```python
from build123d import *

# Parameters (mm, degrees)
EXTRUDE_1_DEPTH                  = 296
CUT_EXTRUDE_1_REACH              = 375.122
SKETCH_2_R                       = 24
EXTRUDE_START                    = -296
EXTRUDE_2_DEPTH                  = 296
CUT_EXTRUDE_2_REACH              = 369.94
CUT_EXTRUDE_2_DIRECTION_2_REACH  = 369.94
SKETCH_5_R                       = 38
CUT_EXTRUDE_4_DEPTH              = 16
CUT_EXTRUDE_4_DIRECTION_2_REACH  = 369.94
CUT_EXTRUDE_10_REACH             = 369.94
CUT_EXTRUDE_11_REACH             = 369.94
CUT_EXTRUDE_12_REACH             = 369.94
CUT_EXTRUDE_12_DIRECTION_2_REACH = 369.94
CUT_EXTRUDE_1_2_DEPTH            = 374.122168517
CUT_EXTRUDE_1_2_DEPTH_BACK       = 6
SKETCH_10_W                      = 353.554121084
SKETCH_10_H                      = 70
CUT_EXTRUDE_2_2_DEPTH            = 374.122168517
CUT_EXTRUDE_2_2_DEPTH_BACK       = 10
SKETCH_11_W                      = 315.319296241
SKETCH_11_H                      = 70
CUT_EXTRUDE_13_DEPTH             = 49.976974814


with BuildPart() as part:
    # 草图1 → 凸台-拉伸1 (new body)
    with BuildSketch(Plane.XY):
        with BuildLine():
            Line((-75.187918949, 11.080471294), (-92, -103))
            Line((-92, -103), (-92, -153))
            Line((-92, -153), (-63, -182))
            Line((-63, -182), (-25.55454992, -183.234465387))
            Line((-25.55454992, -183.234465387), (-23.907851937, -133.284626575))
            Line((-23.907851937, -133.284626575), (27.064456588, -134.965032351))
            Line((27.064456588, -134.965032351), (25.417758605, -184.914871163))
            Line((25.417758605, -184.914871163), (109, -187.67032967))
            Line((109, -187.67032967), (128, -168.67032967))
            Line((128, -168.67032967), (128, -85.67032967))
            Line((128, -85.67032967), (87.212696765, -70.515157246))
            Line((87.212696765, -70.515157246), (75.187918949, 11.080471294))
            ThreePointArc((75.187918949, 11.080471294), (0, 76), (-75.187918949, 11.080471294))
        make_face()
    extrude(amount=EXTRUDE_1_DEPTH)

    # 草图2 → Cut-Extrude 1 (cut, up to next)
    with BuildSketch(Plane.XY.offset(296), mode=Mode.PRIVATE) as cut_extrude_1_sk1:
        Circle(SKETCH_2_R)
    cut_extrude_1_tool1 = extrude(cut_extrude_1_sk1.sketch, amount=-CUT_EXTRUDE_1_REACH, mode=Mode.PRIVATE) & part.part
    add(cut_extrude_1_tool1.solids().sort_by_distance((0, 0, 296))[0], mode=Mode.SUBTRACT)

    # 草图3 → 凸台-拉伸2 (add)
    with BuildSketch(Plane.XY.offset(296).offset(EXTRUDE_START)):
        with BuildLine():
            Line((54, 53.478967828), (54, 166))
            Line((54, 166), (16, 166))
            Line((16, 166), (16, 120))
            Line((16, 120), (-12.175135195, 75.018438287))
            ThreePointArc((-12.175135195, 75.018438287), (23.522691723, 72.268132494), (54, 53.478967828))
        make_face()
    extrude(amount=EXTRUDE_2_DEPTH)

    # 草图4 → Cut-Extrude 2 (cut, up to next)
    with BuildSketch(Plane.ZY.offset(-16), mode=Mode.PRIVATE) as cut_extrude_2_sk1:
        with BuildLine():
            Line((159, 124), (159, 116))
            ThreePointArc((159, 116), (148, 105), (137, 116))
            Line((137, 116), (137, 124))
            ThreePointArc((137, 124), (148, 135), (159, 124))
        make_face()
    cut_extrude_2_tool1 = extrude(cut_extrude_2_sk1.sketch, amount=-CUT_EXTRUDE_2_REACH, mode=Mode.PRIVATE) & part.part
    add(cut_extrude_2_tool1.solids().sort_by_distance((16, 120, 148))[0], mode=Mode.SUBTRACT)

    # 草图4 → Cut-Extrude 2 direction 2 (cut, up to next)
    with BuildSketch(Plane.ZY.offset(-16), mode=Mode.PRIVATE) as cut_extrude_2_direction_2_sk1:
        with BuildLine():
            Line((159, 124), (159, 116))
            ThreePointArc((159, 116), (148, 105), (137, 116))
            Line((137, 116), (137, 124))
            ThreePointArc((137, 124), (148, 135), (159, 124))
        make_face()
    cut_extrude_2_direction_2_tool1 = extrude(cut_extrude_2_direction_2_sk1.sketch, amount=CUT_EXTRUDE_2_DIRECTION_2_REACH, mode=Mode.PRIVATE) & part.part
    add(cut_extrude_2_direction_2_tool1.solids().sort_by_distance((16, 120, 148))[0], mode=Mode.SUBTRACT)

    # 草图5 → 切除-拉伸4 (cut)
    with BuildSketch(Plane.ZY.offset(-16)):
        with Locations((148, 120)):
            Circle(SKETCH_5_R)
    extrude(amount=-CUT_EXTRUDE_4_DEPTH, mode=Mode.SUBTRACT)

    # 草图5 → 切除-拉伸4 direction 2 (cut, up to next)
    with BuildSketch(Plane.ZY.offset(-16), mode=Mode.PRIVATE) as cut_extrude_4_direction_2_sk1:
        with Locations((148, 120)):
            Circle(SKETCH_5_R)
    cut_extrude_4_direction_2_tool1 = extrude(cut_extrude_4_direction_2_sk1.sketch, amount=CUT_EXTRUDE_4_DIRECTION_2_REACH, mode=Mode.PRIVATE) & part.part
    add(cut_extrude_4_direction_2_tool1.solids().sort_by_distance((16, 120, 148))[0], mode=Mode.SUBTRACT)

    # 草图6 → 切除-拉伸10 (cut, up to next)
    with BuildSketch(Plane.ZY.offset(-16), mode=Mode.PRIVATE) as cut_extrude_10_sk1:
        with BuildLine():
            Line((195.958315233, 120), (296, 120))
            Line((296, 120), (296, 166))
            Line((296, 166), (148, 166))
            ThreePointArc((148, 166), (181.226495452, 152.641016151), (195.958315233, 120))
        make_face()
    cut_extrude_10_tool1 = extrude(cut_extrude_10_sk1.sketch, amount=-CUT_EXTRUDE_10_REACH, mode=Mode.PRIVATE) & part.part
    add(cut_extrude_10_tool1.solids().sort_by_distance((16, 144.191812, 240.106882))[0], mode=Mode.SUBTRACT)

    # 草图6<5> → 切除-拉伸11 (cut, up to next)
    with BuildSketch(Plane.ZY.offset(-16), mode=Mode.PRIVATE) as cut_extrude_11_sk1:
        with BuildLine():
            ThreePointArc((100.041684767, 120), (114.773504548, 152.641016151), (148, 166))
            Line((148, 166), (0, 166))
            Line((0, 166), (0, 120))
            Line((0, 120), (100.041684767, 120))
        make_face()
    cut_extrude_11_tool1 = extrude(cut_extrude_11_sk1.sketch, amount=-CUT_EXTRUDE_11_REACH, mode=Mode.PRIVATE) & part.part
    add(cut_extrude_11_tool1.solids().sort_by_distance((16, 144.191812, 55.893118))[0], mode=Mode.SUBTRACT)

    # 草图6<6> → 切除-拉伸12 (cut, up to next)
    with BuildSketch(Plane.ZY.offset(-16), mode=Mode.PRIVATE) as cut_extrude_12_sk1:
        with BuildLine():
            ThreePointArc((100.041684767, 116), (100, 118), (100.041684767, 120))
            Line((100.041684767, 120), (0, 120))
            Line((0, 120), (0, 75.018438287))
            Line((0, 75.018438287), (10, 75.018438287))
            Line((10, 75.018438287), (100.041684767, 116))
        make_face()
    cut_extrude_12_tool1 = extrude(cut_extrude_12_sk1.sketch, amount=-CUT_EXTRUDE_12_REACH, mode=Mode.PRIVATE) & part.part
    # 草图6<6> → 切除-拉伸12 (cut, up to next)
    with BuildSketch(Plane.ZY.offset(-16), mode=Mode.PRIVATE) as cut_extrude_12_sk2:
        with BuildLine():
            Line((286, 75.018438287), (296, 75.018438287))
            Line((296, 75.018438287), (296, 120))
            Line((296, 120), (195.958315233, 120))
            ThreePointArc((195.958315233, 120), (196, 118), (195.958315233, 116))
            Line((195.958315233, 116), (286, 75.018438287))
        make_face()
    cut_extrude_12_tool2 = extrude(cut_extrude_12_sk2.sketch, amount=-CUT_EXTRUDE_12_REACH, mode=Mode.PRIVATE) & part.part
    add(cut_extrude_12_tool1.solids().sort_by_distance((16, 103.644966, 36.114885))[0], mode=Mode.SUBTRACT)
    add(cut_extrude_12_tool2.solids().sort_by_distance((16, 103.644966, 259.885115))[0], mode=Mode.SUBTRACT)

    # 草图6<6> → 切除-拉伸12 direction 2 (cut, up to next)
    with BuildSketch(Plane.ZY.offset(-16), mode=Mode.PRIVATE) as cut_extrude_12_direction_2_sk1:
        with BuildLine():
            ThreePointArc((100.041684767, 116), (100, 118), (100.041684767, 120))
            Line((100.041684767, 120), (0, 120))
            Line((0, 120), (0, 75.018438287))
            Line((0, 75.018438287), (10, 75.018438287))
            Line((10, 75.018438287), (100.041684767, 116))
        make_face()
    cut_extrude_12_direction_2_tool1 = extrude(cut_extrude_12_direction_2_sk1.sketch, amount=CUT_EXTRUDE_12_DIRECTION_2_REACH, mode=Mode.PRIVATE) & part.part
    # 草图6<6> → 切除-拉伸12 direction 2 (cut, up to next)
    with BuildSketch(Plane.ZY.offset(-16), mode=Mode.PRIVATE) as cut_extrude_12_direction_2_sk2:
        with BuildLine():
            Line((286, 75.018438287), (296, 75.018438287))
            Line((296, 75.018438287), (296, 120))
            Line((296, 120), (195.958315233, 120))
            ThreePointArc((195.958315233, 120), (196, 118), (195.958315233, 116))
            Line((195.958315233, 116), (286, 75.018438287))
        make_face()
    cut_extrude_12_direction_2_tool2 = extrude(cut_extrude_12_direction_2_sk2.sketch, amount=CUT_EXTRUDE_12_DIRECTION_2_REACH, mode=Mode.PRIVATE) & part.part
    add(cut_extrude_12_direction_2_tool1.solids().sort_by_distance((16, 103.644966, 36.114885))[0], mode=Mode.SUBTRACT)
    add(cut_extrude_12_direction_2_tool2.solids().sort_by_distance((16, 103.644966, 259.885115))[0], mode=Mode.SUBTRACT)

    # 草图10 → Cut-Extrude 1 2 (cut, two sides: drawn at the far end of the back side and taken through both)
    with BuildSketch(Plane.XY.offset(296).offset(-CUT_EXTRUDE_1_2_DEPTH_BACK)):
        with Locations((35.701307798, -162)):
            Rectangle(SKETCH_10_W, SKETCH_10_H)
    extrude(amount=CUT_EXTRUDE_1_2_DEPTH + CUT_EXTRUDE_1_2_DEPTH_BACK, mode=Mode.SUBTRACT)

    # 草图11 → Cut-Extrude 2 2 (cut, two sides: drawn at the far end of the back side and taken through both)
    with BuildSketch(Plane(origin=(0, 0, 0), x_dir=(-1, 0, 0), z_dir=(0, 0, -1)).offset(-CUT_EXTRUDE_2_2_DEPTH_BACK)):
        with Locations((-8.559302508, -162)):
            Rectangle(SKETCH_11_W, SKETCH_11_H)
    extrude(amount=CUT_EXTRUDE_2_2_DEPTH + CUT_EXTRUDE_2_2_DEPTH_BACK, mode=Mode.SUBTRACT)

    # 草图12 → 切除-拉伸13 (cut)
    with BuildSketch(Plane(origin=(-6.061881785, -183.87708082, 0), x_dir=(0.9994570299138168, -0.032949132854323, 0), z_dir=(-0.032949132854323, -0.9994570299138168, 0))):
        with BuildLine():
            Line((31.496742179, 262.5), (87.843649763, 79.657100204))
            ThreePointArc((87.843649763, 79.657100204), (70.653842384, 47.153092416), (38.149834596, 64.342899796))
            Line((38.149834596, 64.342899796), (31.496742179, 85.931852273))
            Line((31.496742179, 85.931852273), (31.496742179, 262.5))
        make_face()
    extrude(amount=-CUT_EXTRUDE_13_DEPTH, mode=Mode.SUBTRACT)


solid = part.part
```
For this review, take the finished solid that the model builds, in its own axes (mm). A direction names the side the tool comes from. Coordinates: 2 decimals unless noted, no trailing zeros. Order: outer loops, then holes, each group sorted by start corner. A loop starts at its lowest first (then second) coordinate and runs counter-clockwise, first axis right, second up. Notation, with made-up numbers: (-27, 43) - (-11, 43) arc R15 cw to (-11, 48) - close; hole circle Ø2 at (-7.5, -1.75). An arc over 180 degrees is marked (long way). Answer as a JSON object with one key per item and string values. Group by question number.
1. For probe 1 along Y at (x, z) = (26, 148); probe 2 along Z at (x, y) = (-36, -154.5); probe 3 along Y at (x, z) = (0, 235), list the stretches that pass through material, from the lowest coordinate up.
2. The part is to be moulded in two halves that separate along Y. For faces 1 (the flat face through (28.73, 95.22, 54.39)), 2 (the cylindrical face through (43, 105, 148)), 3 (the flat face through (43, 120, 137)), 4 (the flat face through (128, -128, 146)), say which applies: pulls with the +Y half, pulls with the -Y half, needs draft (parallel to the pull), parting line crosses it, or undercut.
3. Clearance check with flat-ended pins moving along their axes: P1, Ø1, axis at y = 45, z = 131.5, coming from the +X side; P2, Ø2.5, axis at x = 47, y = 119.5, coming from the -Z side; P3, Ø4, axis at y = -84.5, z = 127.5, coming from the -X side; P4, Ø1.5, axis at x = -58, y = -39.5, coming from the -Z side. State where each tip first meets the part, or that it passes through.
4. We need section A-A on z = 21.5. State the section outline as (x, y) points, then the cut area to 3 significant figures.
5. For faces 5 (the flat face through (54, 84, 146)), 6 (the cylindrical face through (43, 135, 148)), 7 (the flat face through (41, -157, 290)), list the 3-axis set-ups (+Z, -Z, +X, -X, +Y, -Y) from which the entire face can be reached by the end or side of a thin tool; tool diameter is ignored.
6. We need section C-C on x = 0. State the section outline as (y, z) points, then the cut area to 3 significant figures.
7. We need section D-D on y = 97. State the section outline as (x, z) points.
8. We need section B-B on y = 0. State the section outline as (x, z) points, then the cut area to 3 significant figures.
Final values:
{
 "1": {"probe 1": "-134.93 to 82, 158 to 166", "probe 2": "10 to 290", "probe 3": "-134.07 to -24, 24 to 94.46"},
 "2": {"face 1": "pulls with the +Y half", "face 2": "undercut", "face 3": "undercut", "face 4": "needs draft"},
 "3": {"P1": "x = 61.61", "P2": "z = 100", "P3": "x = -89.57", "P4": "z = 0"},
 "4": {"outline": "(-92, -153) - (-63, -182) - (-25.55, -183.23) - (-23.91, -133.28) - (27.06, -134.97) - (25.42, -184.91) - (109, -187.67) - (128, -168.67) - (128, -85.67) - (87.21, -70.52) - (75.19, 11.08) arc R76 ccw to (54, 53.48) - (54, 80.25) - (-8.9, 80.25) - (-12.18, 75.02) arc R76 ccw to (-75.19, 11.08) - (-92, -103) - close; hole circle Ø48 at (0, 0)", "area": "41,100 mm²"},
 "5": {"face 5": "+Z, -Z, +X, +Y", "face 6": "+X, -X", "face 7": "+Z, +X, -X, -Y"},
 "6": {"outline": "(-134.07, 10) - (-127, 10) - (-127, 0) - (-24, 0) - (-24, 296) - (-127, 296) - (-127, 290) - (-134.07, 290) - close; (24, 0) - (75.02, 0) - (75.02, 10) - (94.46, 52.71) - (94.46, 119.87) arc R38 cw to (94.46, 176.13) - (94.46, 243.29) - (75.02, 286) - (75.02, 296) - (24, 296) - close", "area": "51,600 mm²"},
 "7": {"outline": "(1.59, 58.3) - (54, 58.3) - (54, 237.7) - (1.59, 237.7) - (1.59, 178.25) - (32, 178.25) - (32, 117.75) - (1.59, 117.75) - close"},
 "8": {"outline": "(-76.82, 0) - (-24, 0) - (-24, 296) - (-76.82, 296) - close; (24, 0) - (76.82, 0) - (76.82, 296) - (24, 296) - close", "area": "31,300 mm²"}
}
